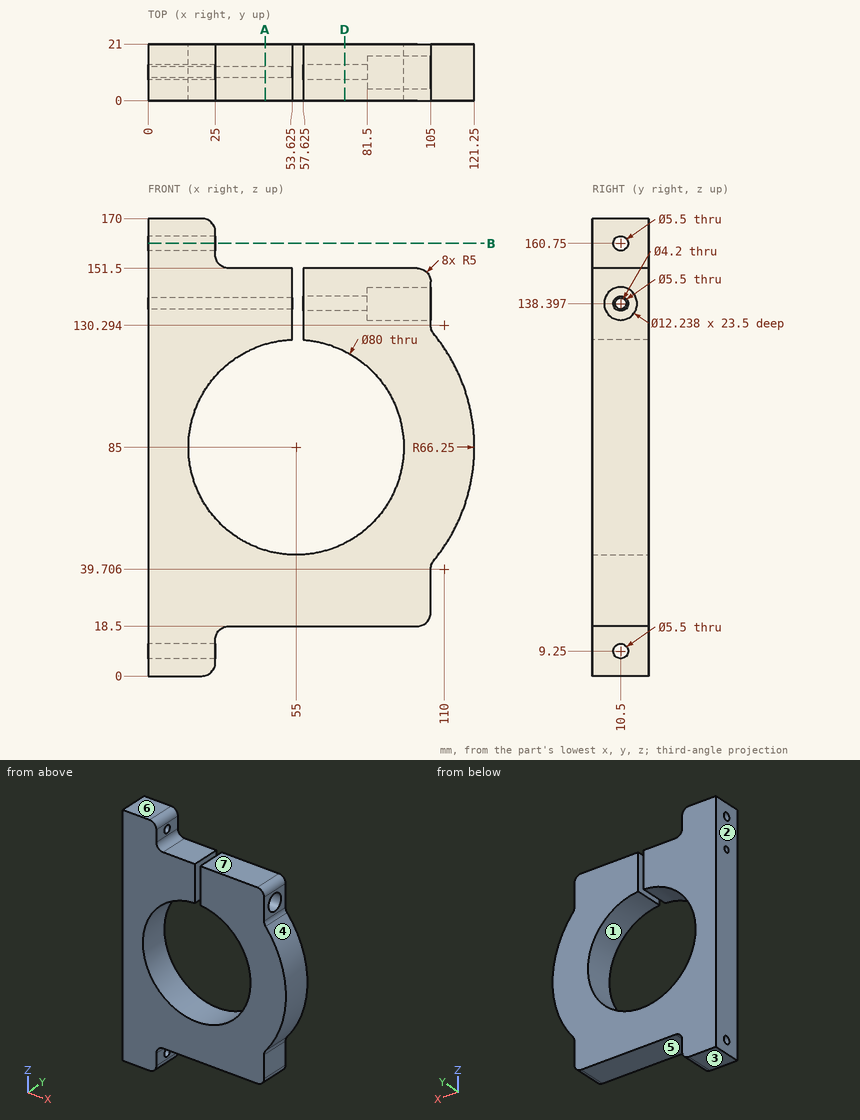
Geometry: see drawing. Coordinates: mm, zero at the bounding-box minimum. A direction names the side the tool comes from. Give positions to 0.01 mm unless a question says otherwise; leave off trailing zeros. Order: outer loops, then holes, each group sorted by start corner. A loop starts at its lowest first (then second) coordinate and runs counter-clockwise, first axis right, second up. Notation, with made-up numbers: (71, 2) -> (119, 2) arc R11 ccw to (119, 8) -> close; hole circle Ø4 at (-34, -27). An arc over 180 degrees is marked (long way). Write each question's results on one line, items separated by ' | '.
1) Cut plane A-A (x = 43.5). Output: boundary loops of the cut face in (y, z), and give its area (3 significant figures).
Geometry says:
outline: (0, 18.5) -> (21, 18.5) -> (21, 46.69) -> (0, 46.69) -> close; (0, 123.31) -> (21, 123.31) -> (21, 151.5) -> (0, 151.5) -> close; hole circle Ø4.2 at (10.5, 138.4) | area: 1,170 mm²
2) Line query: line 1 along Z through (x, y) = (43, 9); line 2 along X through (y, z) = (4.25, 85.5); line 3 along X through (y, z) = (19, 141) (3 decimals). Output: solid intervals per line, ascending.
Geometry says:
line 1: z = 18.5 to 46.84, 123.16 to 136.93, 139.87 to 151.5 | line 2: x = 0 to 15, 95 to 121.25 | line 3: x = 0 to 53.625, 57.625 to 105
3) First-contact query: pin 1 Ø1 at (y, z) = (10, 61.5) entering from +X; pin 2 Ø10.5 at (y, z) = (15, 143) entering from +X; pin 3 Ø5 at (x, y) = (90, 3) entering from +Z; pin 4 Ø2 at (x, z) = (15, 84.5) entering from -Y. Flat tips, straight axial feed; report the tip coordinate or a pass-through.
Geometry says:
pin 1: stops at x = 117.13 | pin 2: stops at x = 105 | pin 3: stops at z = 151.5 | pin 4: stops at y = 0
4) Draft query along X for the marked faces 1, 2, 3 and 4. Return one class per face: released by +X, released by -X, zero draft, split by the parting line, or undercut.
Geometry says:
face 1: undercut | face 2: released by -X | face 3: zero draft | face 4: released by +X
5) Cut plane B-B (z = 160.75). Output: boundary loops of the cut face in (x, y).
Geometry says:
outline: (0, 0) -> (25, 0) -> (25, 7.75) -> (0, 7.75) -> close; (0, 13.25) -> (25, 13.25) -> (25, 21) -> (0, 21) -> close
6) Cut plane D-D (x = 73). Output: boundary loops of the cut face in (y, z).
Geometry says:
outline: (0, 18.5) -> (21, 18.5) -> (21, 49.28) -> (0, 49.28) -> close; (0, 120.72) -> (21, 120.72) -> (21, 151.5) -> (0, 151.5) -> close; hole circle Ø5.5 at (10.5, 138.4)
7) Set-up query: the marked faces 5, 6 and 7. Return all of +Z, -Z, +X, -X, +Y, -Y with unobstructed straight access to the full face (end or side cutting, diameter ignored); none if empty.
Geometry says:
face 5: -Z, +X, +Y, -Y | face 6: +Z, +X, -X, +Y, -Y | face 7: +Z, +X, +Y, -Y
